Source: CAD feature listing. Evaluate the final solid. Frame: model axes, mm. Face numbers are marked on the shaded views. A direction names the side the tool comes from. Give positions to 0.01 mm unless a question says otherwise; leave off trailing zeros. Write each loop counter-clockwise with the first axis right and the second up, starting at its lowest first coordinate (ties: lowest second). Pieces come first, ordered by that corner, then holes. Notation, with made-up numbers: (83, 22.5) - (87, 22.5) arc R18 cw to (87, 34.5) - close; hole circle Ø10 at (-18.75, 77.5). An arc over 180 degrees is marked (long way). One line per question, with ' | ' between items. Start each with the question number.
(1) Ray query, line 1 (Z direction, x = 46.5, y = 23.25); line 2 (Z direction, x = -13, y = 17.5); line 3 (Z direction, x = -46.5, y = 24). Return the intervals inside material, ascending. Write a range as [from, to].
(2) Section C-C, the plane z = 16.5. Return loops of the section in (x, y).
(3) Pin query (flat end, axial travel): pin 1 (5 mm diameter, centred on x = 3, z = -15.5, fed in from +Y); pin 2 (5.5 mm diameter, centred on y = 15, z = -17.5, fed in from +X). Return the tip coordinate at first contact, or that it passes through.
(4) Section A-A, the plane y = 14. Return loops of the section in (x, z), plus the area to 3 significant figures.
(5) Access query for the marked faces 1, 2 and 3. Directions: +Z, -Z, +X, -X, +Y, -Y. A direction counts if a zero-diameter tool reaches every point of the face in a straight line with its end or side. Return the directions, or none.
(6) Draft query along Z for the marked faces 4, 5, 6 and 7. Return one class per face: +Z half, -Z half, draft (parallel to the pull), parting line (faces both ways), or undercut.
(7) Section B-B, the plane x = -31.5. Return loops of the section in (y, z), plus the area to 3 significant figures.
```python
from build123d import *

# Parameters (mm, degrees)
SKETCH1_W                 = 103
SKETCH1_H                 = 52
SKETCH1_W_2               = 83
SKETCH1_H_2               = 42
BOSS_EXTRUDE1_DEPTH       = 30
SKETCH2_W                 = 103
SKETCH2_H                 = 52
BOSS_EXTRUDE2_DEPTH       = 3
SKETCH3_W                 = 10
SKETCH3_H                 = 15
CUT_EXTRUDE1_DEPTH        = 30
F_5_0MM_DOWEL_HOLE1_D     = 5
F_5_0MM_DOWEL_HOLE1_DEPTH = 10
F_5_0MM_DOWEL_HOLE1_TIP   = 1.502151548
FILLET1_R                 = 3


with BuildPart() as part:
    # Sketch1 → Boss-Extrude1 (new body)
    with BuildSketch(Plane(origin=(0, 0, 0), x_dir=(1, 0, 0), z_dir=(0, 1, 0))):
        Rectangle(SKETCH1_W, SKETCH1_H)
        Rectangle(SKETCH1_W_2, SKETCH1_H_2, mode=Mode.SUBTRACT)
    extrude(amount=BOSS_EXTRUDE1_DEPTH)

    # Sketch2 → Boss-Extrude2 (add)
    with BuildSketch(Plane.XZ):
        Rectangle(SKETCH2_W, SKETCH2_H)
    extrude(amount=BOSS_EXTRUDE2_DEPTH)

    # Sketch3 → Cut-Extrude1 (cut)
    with BuildSketch(Plane(origin=(0, 30, 0), x_dir=(1, 0, 0), z_dir=(0, 1, 0))):
        with Locations((46.5, 13.5)):
            Rectangle(SKETCH3_W, SKETCH3_H)
        with Locations((-46.5, 8.5)):
            Rectangle(SKETCH3_W, SKETCH3_H)
    extrude(amount=-CUT_EXTRUDE1_DEPTH, mode=Mode.SUBTRACT)

    # Ø5.0mm Dowel Hole1
    with Locations(Plane(origin=(0, 30, 0), x_dir=(1, 0, 0), z_dir=(0, 1, 0))):
        with Locations((-46.5, 21), (46.5, -21), (-46.5, -21)):
            Hole(F_5_0MM_DOWEL_HOLE1_D / 2, depth=F_5_0MM_DOWEL_HOLE1_DEPTH)
            with Locations((0, 0, -(F_5_0MM_DOWEL_HOLE1_DEPTH + F_5_0MM_DOWEL_HOLE1_TIP / 2))):  # 118° drill point
                Cone(0, F_5_0MM_DOWEL_HOLE1_D / 2, F_5_0MM_DOWEL_HOLE1_TIP, mode=Mode.SUBTRACT)

    # Fillet1
    fillet1_edges = [part.edges().sort_by_distance(p)[0] for p in [
        (51.5, 13.5, 26),
        (-51.5, 13.5, 26),
        (-51.5, 13.5, -26),
        (51.5, 13.5, -26),
    ]]
    fillet(fillet1_edges, radius=FILLET1_R)


solid = part.part
```
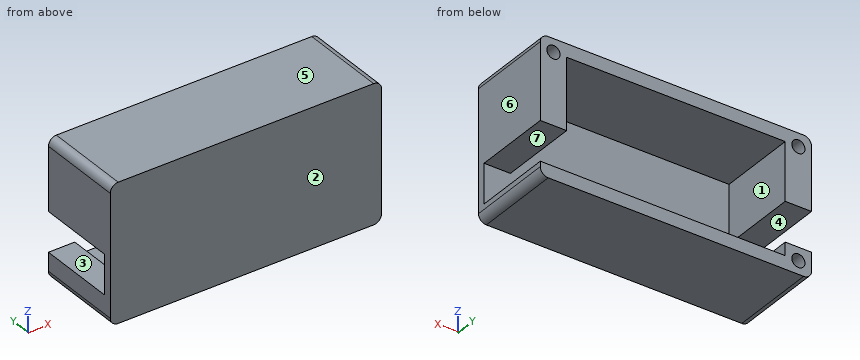
Check sheet entries:
1) line 1: [-26, -21], [-6, 18.5], [23.5, 26] | line 2: [-26, -21], [21, 26] | line 3: [-26, -23.5], [-18.5, -16], [-1, 18.5], [23.5, 26]
2) outline: (-51.5, -3) - (51.5, -3) - (51.5, 30) - (41.5, 30) - (41.5, 0) - (-41.5, 0) - (-41.5, 30) - (-51.5, 30) - close
3) pin 1: y = 0 | pin 2: x = -41.5
4) outline: (-51.5, -23) arc R3 ccw to (-48.5, -26) - (48.5, -26) arc R3 ccw to (51.5, -23) - (51.5, -21) - (-41.5, -21) - (-41.5, -16) - (-51.5, -16) - close; (-51.5, -1) - (-41.5, -1) - (-41.5, 21) - (41.5, 21) - (41.5, -6) - (51.5, -6) - (51.5, 23) arc R3 ccw to (48.5, 26) - (-48.5, 26) arc R3 ccw to (-51.5, 23) - close | area: 1,560 mm²
5) face 1: +Y | face 2: +Z, -Z, +X, -X, -Y | face 3: +X, -X, +Y
6) face 4: undercut | face 5: +Z half | face 6: draft | face 7: undercut
7) outline: (-3, -26) - (30, -26) - (30, -21) - (0, -21) - (0, 21) - (30, 21) - (30, 26) - (-3, 26) - close | area: 456 mm²
